from build123d import *

# Parameters (mm, degrees)
BOSS_EXTRUDE1_DEPTH     = 1.5875
F_1_4_CLEARANCE_HOLE1_D = 6.5278
FILLET1_R               = 6.35
CHAMFER1_SIZE           = 0.254


with BuildPart() as part:
    # Sketch1 → Boss-Extrude1 (new, symmetric)
    with BuildSketch(Plane(origin=(0, 0, 0), x_dir=(0, 0, -1), z_dir=(1, 0, 0))):
        Polygon((0, 127), (-19.05, 127), (-127, 19.05), (-127, 0), (-76.2, 0), (0, 76.2), align=None)
    extrude(amount=BOSS_EXTRUDE1_DEPTH, both=True)

    # 1/4 Clearance Hole1 (through all)
    with Locations(Plane(origin=(1.5875, 0, 0), x_dir=(0, 0, -1), z_dir=(1, 0, 0))):
        with Locations((-114.3, 9.525), (-88.9, 9.525), (-9.525, 88.9), (-9.525, 114.3)):
            Hole(F_1_4_CLEARANCE_HOLE1_D / 2)

    # Fillet1
    fillet1_edges = [part.edges().sort_by_distance(p)[0] for p in [
        (0, 76.2, 0),
        (0, 0, 76.2),
        (0, 0, 127),
        (0, 19.05, 127),
        (0, 127, 19.05),
        (0, 127, 0),
    ]]
    fillet(fillet1_edges, radius=FILLET1_R)

    # Chamfer1
    chamfer1_edges = [part.edges().sort_by_distance(p)[0] for p in [
        (1.5875, 114.3, 6.2611),
        (-1.5875, 114.3, 6.2611),
        (1.5875, 88.9, 6.2611),
        (-1.5875, 88.9, 6.2611),
        (1.5875, 9.525, 85.6361),
        (-1.5875, 9.525, 85.6361),
        (1.5875, 9.525, 111.0361),
        (-1.5875, 9.525, 111.0361),
    ]]
    chamfer(chamfer1_edges, length=CHAMFER1_SIZE)


solid = part.part
Can you work these out from the model? Positions are in its coordinate system, mm. Give positions to 0.01 mm unless a question says otherwise; leave off trailing zeros. Loops run counter-clockwise (first coordinate to the right, second up) from the corner with the lowest first, then second, coordinate; pieces in that order, holes last. Notation, with made-up numbers: (-3.5, -16) -> (26.5, -16) arc R30 cw to (26.5, 7) -> close; hole circle Ø5 at (-25, -26.75). An arc over 180 degrees is marked (long way). Return JSON: item names as keys, results as strings.
Q1. I want a section at A-A, the plane z = 88.9. List the corners of the cut face in (x, y) for me.
Checks:
{"outline": "(-1.59, 0) -> (1.59, 0) -> (1.59, 6.01) -> (1.33, 6.26) -> (-1.33, 6.26) -> (-1.59, 6.01) -> close; (-1.59, 13.04) -> (-1.33, 12.79) -> (1.33, 12.79) -> (1.59, 13.04) -> (1.59, 57.15) -> (-1.59, 57.15) -> close"}
Q2. We'd pull the mould along Z, two halves only. Please class faces 1 (the face through (-0.02, 9.67, 85.64)), 2 (the face through (0, 0, 100)), 3 (the face through (0, 99, 0)): released by +Z, released by -Z, zero draft, split by the parting line, or undercut.
Checks:
{"face 1": "undercut", "face 2": "zero draft", "face 3": "released by -Z"}
Q3. For pin 1 Ø1 at (x, z) = (0.5, 74) entering from +Y, with a flat end and sliding along its axis, tell me the tip position at first contact or that it passes through.
Checks:
{"pin 1": "stops at y = 72.55"}
Q4. I want a section at D-D, the plane y = 103.5. List the corners of the cut face in (x, z) for me.
Checks:
{"outline": "(-1.59, 0) -> (1.59, 0) -> (1.59, 42.55) -> (-1.59, 42.55) -> close"}
Q5. I need wall thicknesses on probe 1 along Y at (x, z) = (0.4, 8.5); probe 2 along Y at (x, z) = (0.85, 9); probe 3 along Y at (x, z) = (-0.35, 114.3). Which ranges of each line are inside material? Lowest first, please.
Checks:
{"probe 1": "y = 67.7 to 85.8, 92 to 111.2, 117.4 to 127", "probe 2": "y = 67.2 to 85.68, 92.12 to 111.08, 117.52 to 127", "probe 3": "y = 0 to 6.26, 12.79 to 31.75"}
Q6. I want a section at C-C, the plane x = 0.15. List the corners of the cut face in (y, z) for me (3 decimals).
Checks:
{"outline": "(0, 78.83) arc R6.35 ccw to (1.86, 74.34) -> (74.34, 1.86) arc R6.35 ccw to (78.83, 0) -> (120.65, 0) arc R6.35 ccw to (127, 6.35) -> (127, 16.42) arc R6.35 ccw to (125.14, 20.91) -> (20.91, 125.14) arc R6.35 ccw to (16.42, 127) -> (6.35, 127) arc R6.35 ccw to (0, 120.65) -> close; hole circle Ø6.528 at (9.525, 88.9); hole circle Ø6.528 at (9.525, 114.3); hole circle Ø6.528 at (88.9, 9.525); hole circle Ø6.528 at (114.3, 9.525)"}
